For this review, take the finished solid that the model builds, in its own axes (mm). A direction names the side the tool comes from. Round coordinates to 2 decimals unless told otherwise and drop trailing zeros. Write each loop counter-clockwise with the first axis right and the second up, starting at its lowest first coordinate (ties: lowest second). Pieces come first, ordered by that corner, then holes. Notation, with made-up numbers: (89, -21.5) -> (122, -21.5) arc R24 cw to (122, 5.5) -> close; hole circle Ø4 at (48, 14). An arc over 180 degrees is marked (long way). Write each question's results on one line, items separated by ' | '. Start each with the question number.
Item 1: To check wall thickness, follow line 1 along X through (y, z) = (22, 0); line 2 along Y through (x, z) = (0, 11.5); line 3 along X through (y, z) = (20.5, 6). State the ranges of each line that lie inside material, in increasing order.
Item 2: Add section A-A (y = 18.5). State the section outline as (x, z) points, plus the area to 3 significant figures.
Item 3: The part is to be moulded in two halves that separate along X. For faces 1 (the flat face through (7.5, 34, 26)), 2 (the cylindrical face through (21.78, 19.75, 69.15)), 3 (the flat face through (-15, 40, -48)), say which applies: +X half, -X half, draft (parallel to the pull), parting line (faces both ways), or undercut.
Item 4: Tool access review of faces 4 (the flat face through (26, 0, -40)), 5 (the cylindrical face through (0, 21, 10)), 6 (the flat face through (-26, 30, 15)): name each direction out of +Z, -Z, +X, -X, +Y, -Y from which nothing blocks a thin tool from reaching the whole face with its end or side.
Item 5: Clearance check with flat-ended pins moving along their axes: pin 1 (10 mm diameter, centred on y = 23, z = 14, fed in from +X); pin 2 (12 mm diameter, centred on y = 6.5, z = -32.5, fed in from +X); pin 3 (3 mm diameter, centred on y = 36, z = -29.5, fed in from +X); pin 4 (6 mm diameter, centred on x = 0, z = 0, fed in from -Y). State where each tip first meets the part, or that it passes through.
Item 6: Add section B-B (y = 28). State the section outline as (x, z) points, plus the area to 3 significant figures.
from build123d import *

# Parameters (mm, degrees)
SKETCH1_R             = 50
SKETCH1_R_2           = 47.5
BOSS_EXTRUDE1_DEPTH   = 40
SKETCH1_R_3           = 15
SKETCH1_R_4           = 5
BOSS_EXTRUDE1_2_DEPTH = 40
BOSS_EXTRUDE2_DEPTH   = 7.5
CIRPATTERN1_COUNT     = 6
FILLET1_R             = 1
SKETCH5_R             = 72.5
SKETCH5_R_2           = 50
BOSS_EXTRUDE4_DEPTH   = 40
FILLET2_R             = 2
FILLET3_R             = 0.1
SKETCH7_R             = 15
CUT_EXTRUDE1_DEPTH    = 10
SKETCH8_R             = 2.5
CUT_EXTRUDE2_DEPTH    = 17.5


with BuildPart() as part:
    # Sketch1 → Boss-Extrude1 (new body)
    with BuildSketch(Plane(origin=(0, 0, 0), x_dir=(1, 0, 0), z_dir=(0, 1, 0))):
        with Locations(Location((0, 0, 0), (0, 0, 270))):
            Circle(SKETCH1_R)
        with Locations(Location((0, 0, 0), (0, 0, 270))):
            Circle(SKETCH1_R_2, mode=Mode.SUBTRACT)
    extrude(amount=BOSS_EXTRUDE1_DEPTH)

    # Sketch2 → Boss-Extrude2 (add, symmetric)
    with BuildSketch(Plane(origin=(0, 0, 0), x_dir=(0, 0, -1), z_dir=(1, 0, 0))):
        with BuildLine():
            Line((48.889169482, 30), (8.889169482, 30))
            Line((8.889169482, 30), (8.889169482, 40))
            add(Edge.make_bspline(
                [(8.889169482, 40), (29.868778493, 39.876907844), (48.889169482, 30)],
                knots=[0, 0, 0, 1, 1, 1], degree=2))
        make_face()
    boss_extrude2 = extrude(amount=BOSS_EXTRUDE2_DEPTH, both=True)

    # CirPattern1: Boss-Extrude2 ×6 about axis
    cirpattern1_axis = Axis((0, 40, 0), (0, 1, 0))
    for i in range(1, CIRPATTERN1_COUNT):
        add(boss_extrude2.rotate(cirpattern1_axis, i * 360 / CIRPATTERN1_COUNT))

    # Fillet1
    fillet1_edges = [part.edges().sort_by_distance(p)[0] for p in [
        (0, 40, -50),
        (0, 0, -50),
    ]]
    fillet(fillet1_edges, radius=FILLET1_R)


with BuildPart() as body_2:
    # Sketch1 → Boss-Extrude1 2 (new body)
    with BuildSketch(Plane(origin=(0, 0, 0), x_dir=(1, 0, 0), z_dir=(0, 1, 0))):
        with Locations(Location((0, 0, 0), (0, 0, 270))):
            Circle(SKETCH1_R_3)
        with Locations(Location((0, 0, 0), (0, 0, 270))):
            Circle(SKETCH1_R_4, mode=Mode.SUBTRACT)
    extrude(amount=BOSS_EXTRUDE1_2_DEPTH)


    add(part.part)  # Boss-Extrude4 merges part
    # Sketch5 → Boss-Extrude4 (add)
    with BuildSketch(Plane(origin=(0, 0, 0), x_dir=(1, 0, 0), z_dir=(0, 1, 0))):
        with Locations(Location((0, 0, 0), (0, 0, 270))):
            Circle(SKETCH5_R)
        with Locations(Location((0, 0, 0), (0, 0, 270))):
            Circle(SKETCH5_R_2, mode=Mode.SUBTRACT)
    extrude(amount=BOSS_EXTRUDE4_DEPTH)

    # Fillet2
    fillet2_edges = [body_2.edges().sort_by_distance(p)[0] for p in [
        (0, 40, -72.5),
        (0, 0, -72.5),
    ]]
    fillet(fillet2_edges, radius=FILLET2_R)

    # Fillet3
    fillet3_edges = [body_2.edges().sort_by_distance(p)[0] for p in [
        (0, 40, -50),
    ]]
    fillet(fillet3_edges, radius=FILLET3_R)

    # Sketch7 → Cut-Extrude1 (cut)
    with BuildSketch(Plane.XZ):
        with Locations(Location((0, 0, 0), (0, 0, 270))):
            Circle(SKETCH7_R)
    extrude(amount=-CUT_EXTRUDE1_DEPTH, mode=Mode.SUBTRACT)

    # Sketch8 → Cut-Extrude2 (cut, symmetric)
    with BuildSketch(Plane.XY):
        with Locations((0, 18.5)):
            Circle(SKETCH8_R)
    extrude(amount=CUT_EXTRUDE2_DEPTH, both=True, mode=Mode.SUBTRACT)


solid = body_2.part
Responses:
1) line 1: x = -72.5 to -47.5, -15 to -5, 5 to 15, 47.5 to 72.5 | line 2: y = 10 to 16, 21 to 40 | line 3: x = -72.25 to -47.12, -13.75 to -1.5, 1.5 to 13.75, 47.12 to 72.25
2) outline: circle Ø145 at (0, 0); (-2.5, -14.79) -> (-2.5, -4.33) arc R5 cw to (-2.5, 4.33) -> (-2.5, 14.79) arc R15 ccw to start; (2.5, -14.79) arc R15 ccw to (2.5, 14.79) -> (2.5, 4.33) arc R5 cw to (2.5, -4.33) -> close; hole circle Ø95 at (0, 0) | area: 9,950 mm^2
3) face 1: undercut | face 2: parting line | face 3: draft
4) face 4: +Z, -Z, +X, -X, -Y | face 5: none | face 6: -Y
5) pin 1: stops at x = 71.94 | pin 2: stops at x = 67.48 | pin 3: stops at x = 66.87 | pin 4: passes through
6) outline: circle Ø145 at (0, 0); circle Ø30 at (0, 0); hole circle Ø95 at (0, 0); hole circle Ø10 at (0, 0) | area: 10,100 mm^2
